from build123d import *

# Parameters (mm, degrees)
SKETCH_R        = 30
PAD_DEPTH       = 6
SKETCH006_R     = 29
POCKET_DEPTH    = 1
SKETCH007_W     = 10
SKETCH007_H     = 9.5
PAD001_DEPTH    = 5
SKETCH002_R     = 12
PAD002_DEPTH    = 6
SKETCH003_R     = 11
POCKET001_DEPTH = 1
SKETCH004_R     = 10
POCKET002_DEPTH = 4
POCKET003_DEPTH = 2


with BuildPart() as part:
    # Sketch → Pad (new body)
    with BuildSketch(Plane.XY):
        Circle(SKETCH_R)
    extrude(amount=PAD_DEPTH)

    # Sketch006 (on Face3 of Pad) → Pocket (cut)
    with BuildSketch(Plane.XY.offset(6)):
        Circle(SKETCH006_R)
    extrude(amount=-POCKET_DEPTH, mode=Mode.SUBTRACT)

    # Sketch007 → Pad001 (join)
    with BuildSketch(Plane.XY):
        with Locations((0, -34.330399)):
            Rectangle(SKETCH007_W, SKETCH007_H)
    extrude(amount=PAD001_DEPTH)

    # Sketch002 → Pad002 (join)
    with BuildSketch(Plane.XY):
        with Locations((24, -18)):
            Circle(SKETCH002_R)
    extrude(amount=PAD002_DEPTH)

    # Sketch003 (on Face14 of Pad002) → Pocket001 (cut)
    with BuildSketch(Plane.XY.offset(6)):
        with Locations((24, -18)):
            Circle(SKETCH003_R)
    extrude(amount=-POCKET001_DEPTH, mode=Mode.SUBTRACT)

    # Sketch004 (on Face24 of Pocket001) → Pocket002 (cut)
    with BuildSketch(Plane.XY.offset(5)):
        with Locations((24, -18)):
            Circle(SKETCH004_R)
    extrude(amount=-POCKET002_DEPTH, mode=Mode.SUBTRACT)

    # Sketch005 → Pocket003 (cut)
    with BuildSketch(Plane(origin=(0, 0, 0), x_dir=(1, 0, 0), z_dir=(0, 0, -1))):
        Polygon((13.091288, 23), (24, 23), (24, 13), (13.091288, 13), (13.091288, 16), (0, 16), (-2, 16), (-2, 34.580399), (2, 34.580399), (2, 20), (13.091288, 20), align=None)
    extrude(amount=-POCKET003_DEPTH, mode=Mode.SUBTRACT)


solid = part.part
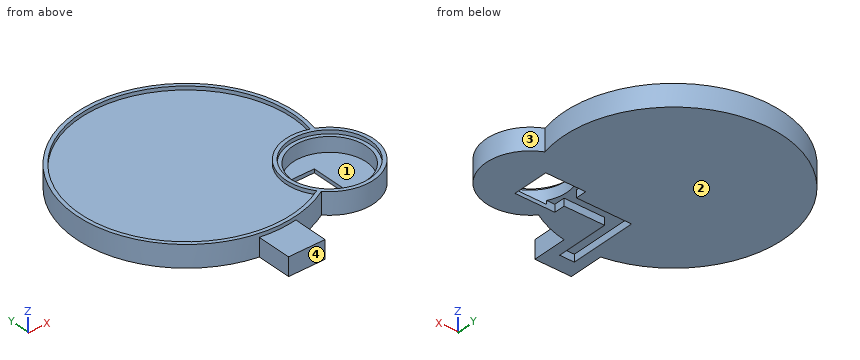
Part model, mm, in its own coordinate system. Face numbers are marked on the shaded views. A direction names the side the tool comes from. Give positions to 0.01 mm unless a question says otherwise; leave off trailing zeros. Order: outer loops, then holes, each group sorted by start corner. A loop starts at its lowest first (then second) coordinate and runs counter-clockwise, first axis right, second up. Notation, with made-up numbers: (6, -36) - (41, -36) arc R21 cw to (41, -26) - close; hole circle Ø7 at (70, -18.75). An arc over 180 degrees is marked (long way). Use a Markdown table: item, result.
1) 3-axis set-ups, long thin cutter, end or side, ignore diameter. For the marked faces 1 and 2: which of +Z, -Z, +X, -X, +Y, -Y reach the whole face in a straight line?
Checked values:
| item | result |
|---|---|
| face 1 | +Z |
| face 2 | -Z, +X, -X, +Y, -Y |
2) Saw through at D-D on y = -18. List the corners of the cut face in (x, z).
Checked values:
| item | result |
|---|---|
| outline | (-24, 0) - (-2, 0) - (-2, 2) - (14, 2) - (14, 5) - (13, 5) - (13, 6) - (12, 6) - (12, 5) - (-22.74, 5) - (-22.74, 6) - (-24, 6) - close; (24, 0) - (36, 0) - (36, 6) - (35, 6) - (35, 5) - (34, 5) - (34, 1) - (24, 1) - close |
3) Saw through at A-A on y = 0. List the corners of the cut face in (x, z).
Checked values:
| item | result |
|---|---|
| outline | (-30, 0) - (30, 0) - (30, 6) - (29, 6) - (29, 5) - (-29, 5) - (-29, 6) - (-30, 6) - close |
4) Probe L1, parallel to Y at x = 0, z = 5.45; L2, parallel to X at y = -9.5, z = 5.85. List the from-to ranges inside material, lowest first. Write a range as from..to.
Checked values:
| item | result |
|---|---|
| L1 | -30..-29, 29..30 |
| L2 | -28.46..-27.4, 15.53..17.02, 30.98..32.47 |
5) Flat gauge pins, fed straight in: P1, Ø0.6, axis at x = 16.5, z = 0.5, coming from the -Y side; P2, Ø4, axis at x = -21.5, y = -21, coming from the +Z side; P3, Ø3, axis at y = -22.5, z = 1.5, coming from the +X side; P4, Ø0.5, axis at y = -20.5, z = 0.5, coming from the -X side. Where does each tip first touch, or does it go through?
Checked values:
| item | result |
|---|---|
| P1 | y = -27.6 |
| P2 | z = 6 |
| P3 | x = 35.62 |
| P4 | x = -22.13 |
6) Two-plate mould, pull along X, no slides. Class the marked faces 3 and 4: +X half, -X half, draft (parallel to the pull), parting line (faces both ways), or undercut.
Checked values:
| item | result |
|---|---|
| face 3 | undercut |
| face 4 | draft |
7) Saw through at B-B on x = 0. List the corners of the cut face in (y, z).
Checked values:
| item | result |
|---|---|
| outline | (-39.08, 0) - (-34.58, 0) - (-34.58, 2) - (-16, 2) - (-16, 0) - (30, 0) - (30, 6) - (29, 6) - (29, 5) - (-29, 5) - (-29, 6) - (-30, 6) - (-30, 5) - (-39.08, 5) - close |
8) Saw through at C-C on z = 3. List the corners of the cut face in (x, y).
Checked values:
| item | result |
|---|---|
| outline | (-5, -39.08) - (5, -39.08) - (5, -29.58) arc R30 ccw to (15.03, -25.97) arc R12 ccw (long way) to (29.13, -7.15) arc R30 ccw (long way) to (-5, -29.58) - close; hole circle Ø20 at (24, -18) |
